from build123d import *

# Parameters (mm, degrees)
SKETCH1_W           = 65
SKETCH1_H           = 15
BOSS_EXTRUDE1_DEPTH = 4
SKETCH2_W           = 45
SKETCH2_H           = 15
BOSS_EXTRUDE2_DEPTH = 56
SKETCH3_R           = 5
CUT_EXTRUDE1_DEPTH  = 10
CUT_EXTRUDE5_REACH  = 17
BOSS_EXTRUDE3_DEPTH = 10
CUT_EXTRUDE6_REACH  = 6
SKETCH8_R           = 1.5
CUT_EXTRUDE7_DEPTH  = 22.5
SKETCH10_R          = 1.6
BOSS_EXTRUDE4_DEPTH = 20
SKETCH11_R          = 1.6
CUT_EXTRUDE8_DEPTH  = 35
SKETCH12_R          = 2.5
SKETCH12_R_2        = 1.6
BOSS_EXTRUDE5_DEPTH = 1


with BuildPart() as part:
    # Sketch1 → Boss-Extrude1 (new body)
    with BuildSketch(Plane(origin=(0, 0, 0), x_dir=(1, 0, 0), z_dir=(0, 1, 0))):
        Rectangle(SKETCH1_W, SKETCH1_H)
    extrude(amount=BOSS_EXTRUDE1_DEPTH)

    # Sketch2 → Boss-Extrude2 (add)
    with BuildSketch(Plane(origin=(0, 4, 0), x_dir=(1, 0, 0), z_dir=(0, 1, 0))):
        Rectangle(SKETCH2_W, SKETCH2_H)
    extrude(amount=BOSS_EXTRUDE2_DEPTH)

    # Sketch3 → Cut-Extrude1 (cut)
    with BuildSketch(Plane.XY.offset(7.5)):
        with Locations((0, 51)):
            Circle(SKETCH3_R)
    extrude(amount=-CUT_EXTRUDE1_DEPTH, mode=Mode.SUBTRACT)

    # Sketch6 → Cut-Extrude5 (cut, up to next)
    with BuildSketch(Plane.XY.offset(7.5), mode=Mode.PRIVATE) as cut_extrude5_sk1:
        with BuildLine():
            Line((5, 60), (22.5, 60))
            Line((22.5, 60), (22.5, 42.5))
            ThreePointArc((22.5, 42.5), (17.374368671, 54.874368671), (5, 60))
        make_face()
    cut_extrude5_tool1 = extrude(cut_extrude5_sk1.sketch, amount=-CUT_EXTRUDE5_REACH, mode=Mode.PRIVATE) & part.part
    add(cut_extrude5_tool1.solids().sort_by_distance((18.591061, 56.091061, 7.5))[0], mode=Mode.SUBTRACT)
    # Sketch6 → Cut-Extrude5 (cut, up to next)
    with BuildSketch(Plane.XY.offset(7.5), mode=Mode.PRIVATE) as cut_extrude5_sk2:
        with BuildLine():
            Line((-22.5, 42.5), (-22.5, 60))
            Line((-22.5, 60), (-5, 60))
            ThreePointArc((-5, 60), (-17.374368671, 54.874368671), (-22.5, 42.5))
        make_face()
    cut_extrude5_tool2 = extrude(cut_extrude5_sk2.sketch, amount=-CUT_EXTRUDE5_REACH, mode=Mode.PRIVATE) & part.part
    add(cut_extrude5_tool2.solids().sort_by_distance((-18.591061, 56.091061, 7.5))[0], mode=Mode.SUBTRACT)

    # Sketch7 → Boss-Extrude3 (add)
    with BuildSketch(Plane(origin=(0, 0, -7.5), x_dir=(-1, 0, 0), z_dir=(0, 0, -1))):
        with BuildLine():
            Line((-22.5, 42.5), (-22.5, 4))
            Line((-22.5, 4), (-32.5, 4))
            Line((-32.5, 4), (-32.5, 0))
            Line((-32.5, 0), (32.5, 0))
            Line((32.5, 0), (32.5, 4))
            Line((32.5, 4), (22.5, 4))
            Line((22.5, 4), (22.5, 42.5))
            ThreePointArc((22.5, 42.5), (17.374368671, 54.874368671), (5, 60))
            Line((5, 60), (-5, 60))
            ThreePointArc((-5, 60), (-17.374368671, 54.874368671), (-22.5, 42.5))
        make_face()
    extrude(amount=BOSS_EXTRUDE3_DEPTH)

    # Sketch8 → Cut-Extrude6 (cut, up to next)
    with BuildSketch(Plane(origin=(0, 4, 0), x_dir=(1, 0, 0), z_dir=(0, 1, 0)), mode=Mode.PRIVATE) as cut_extrude6_sk1:
        with Locations((-27.5, -2.5)):
            Circle(SKETCH8_R)
    cut_extrude6_tool1 = extrude(cut_extrude6_sk1.sketch, amount=-CUT_EXTRUDE6_REACH, mode=Mode.PRIVATE) & part.part
    add(cut_extrude6_tool1.solids().sort_by_distance((-27.5, 4, 2.5))[0], mode=Mode.SUBTRACT)
    # Sketch8 → Cut-Extrude6 (cut, up to next)
    with BuildSketch(Plane(origin=(0, 4, 0), x_dir=(1, 0, 0), z_dir=(0, 1, 0)), mode=Mode.PRIVATE) as cut_extrude6_sk2:
        with Locations((-27.5, 12.5)):
            Circle(SKETCH8_R)
    cut_extrude6_tool2 = extrude(cut_extrude6_sk2.sketch, amount=-CUT_EXTRUDE6_REACH, mode=Mode.PRIVATE) & part.part
    add(cut_extrude6_tool2.solids().sort_by_distance((-27.5, 4, -12.5))[0], mode=Mode.SUBTRACT)
    # Sketch8 → Cut-Extrude6 (cut, up to next)
    with BuildSketch(Plane(origin=(0, 4, 0), x_dir=(1, 0, 0), z_dir=(0, 1, 0)), mode=Mode.PRIVATE) as cut_extrude6_sk3:
        with Locations((27.5, 12.5)):
            Circle(SKETCH8_R)
    cut_extrude6_tool3 = extrude(cut_extrude6_sk3.sketch, amount=-CUT_EXTRUDE6_REACH, mode=Mode.PRIVATE) & part.part
    add(cut_extrude6_tool3.solids().sort_by_distance((27.5, 4, -12.5))[0], mode=Mode.SUBTRACT)
    # Sketch8 → Cut-Extrude6 (cut, up to next)
    with BuildSketch(Plane(origin=(0, 4, 0), x_dir=(1, 0, 0), z_dir=(0, 1, 0)), mode=Mode.PRIVATE) as cut_extrude6_sk4:
        with Locations((27.5, -2.5)):
            Circle(SKETCH8_R)
    cut_extrude6_tool4 = extrude(cut_extrude6_sk4.sketch, amount=-CUT_EXTRUDE6_REACH, mode=Mode.PRIVATE) & part.part
    add(cut_extrude6_tool4.solids().sort_by_distance((27.5, 4, 2.5))[0], mode=Mode.SUBTRACT)

    # Sketch9 → Cut-Extrude7 (cut)
    with BuildSketch(Plane(origin=(0, 60, 0), x_dir=(1, 0, 0), z_dir=(0, 1, 0))):
        Polygon((-2.875, 11.659882024), (-2.875, 17.5), (2.875, 17.5), (2.875, 11.659882024), (2.875, 8.340117976), (0, 6.680235952), (-2.875, 8.340117976), align=None)
    extrude(amount=-CUT_EXTRUDE7_DEPTH, mode=Mode.SUBTRACT)

    # Sketch10 → Boss-Extrude4 (add)
    with BuildSketch(Plane(origin=(0, 60, 0), x_dir=(1, 0, 0), z_dir=(0, 1, 0))):
        Polygon((0, 6.680235952), (2.875, 8.340117976), (2.875, 17.5), (-2.875, 17.5), (-2.875, 8.340117976), align=None)
        with Locations((0, 10)):
            Circle(SKETCH10_R, mode=Mode.SUBTRACT)
    extrude(amount=-BOSS_EXTRUDE4_DEPTH)

    # Sketch11 → Cut-Extrude8 (cut)
    with BuildSketch(Plane(origin=(0, 60, 0), x_dir=(1, 0, 0), z_dir=(0, 1, 0))):
        with Locations((0, 10)):
            Circle(SKETCH11_R)
    extrude(amount=-CUT_EXTRUDE8_DEPTH, mode=Mode.SUBTRACT)

    # Sketch12 → Boss-Extrude5 (add)
    with BuildSketch(Plane(origin=(0, 60, 0), x_dir=(1, 0, 0), z_dir=(0, 1, 0))):
        with Locations((0, 10)):
            Circle(SKETCH12_R)
        with Locations((0, 10)):
            Circle(SKETCH12_R_2, mode=Mode.SUBTRACT)
    extrude(amount=BOSS_EXTRUDE5_DEPTH)


solid = part.part
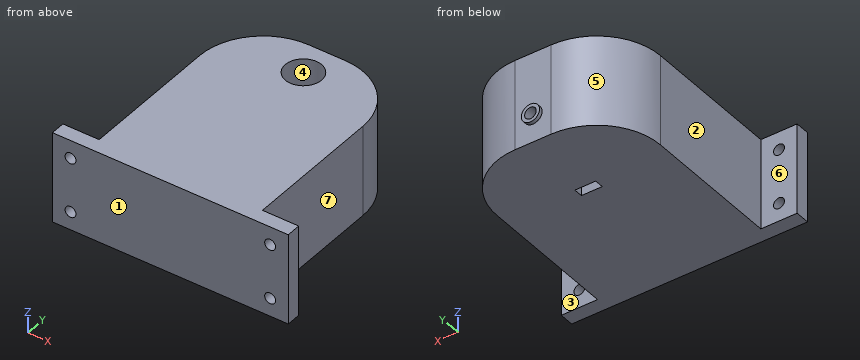
Geometry: final body of the model. Coordinates: model frame, mm. Face numbers are marked on the shaded views. A direction names the side the tool comes from. Coordinates: 2 decimals unless noted, no trailing zeros. Order: outer loops, then holes, each group sorted by start corner. A loop starts at its lowest first (then second) coordinate and runs counter-clockwise, first axis right, second up.
(1) Section query A-A (z = 2.5). Return the cut outline in (x, y).
(2) Section query D-D (z = -10). Return the cut outline in (x, y) (3 decimals), plus the area to 3 significant figures.
(3) Section query B-B (x = -27.5). Return the cut outline in (y, z), plus the area to 3 significant figures.
(4) Section query C-C (y = 51). Return the cut outline in (x, z), plus the area to 3 significant figures.
(5) Material intervals for probe 1 along Z at (x, y) = (27.5, 3.15); probe 2 along X at (y, z) = (2.45, -12.5); probe 3 along Y at (x, z) = (-0.5, -14.25), sorted ascending.
(6) Access query for the marked faces 1, 2 and 3. Directions: +Z, -Z, +X, -X, +Y, -Y. A direction counts if a zero-diameter tool reaches every point of the face in a straight line with its end or side. Return the directions, or none.
(7) First-contact query: pin 1 (4 mm diameter, centred on x = 27.5, z = -12.5, fed in from +Y); pin 2 (6 mm diameter, centred on x = -6.5, z = 2.5, fed in from +Y); pin 3 (11 mm diameter, centred on x = -25.5, z = -8, fed in from +Y). Flat tips, straight axial feed; report the tip coordinate or a pass-through.
(8) Draft query along X for the marked faces 4, 5, 6 and 7. Return one class per face: pulls with the +X half, pulls with the -X half, needs draft (parallel to the pull), parting line crosses it, or undercut.
Solution:
1. outline: (-32.5, 0) - (-29, 0) - (-29, 4) - (-32.5, 4) - close; (-26, 0) - (26, 0) - (26, 4) - (22.5, 4) - (22.5, 42.5) arc R17.5 ccw to (5, 60) - (-5, 60) arc R17.5 ccw to (-22.5, 42.5) - (-22.5, 4) - (-26, 4) - close; (29, 0) - (32.5, 0) - (32.5, 4) - (29, 4) - close; hole circle Ø10 at (0, 51)
2. outline: (-32.5, 0) - (32.5, 0) - (32.5, 4) - (22.5, 4) - (22.5, 42.5) arc R17.5 ccw to (5, 60) - (2.5, 60) - (2.5, 61) - (1.6, 61) - (1.6, 40) - (2.875, 40) - (2.875, 37.5) - (1.6, 37.5) - (1.6, 25) - (-1.6, 25) - (-1.6, 37.5) - (-2.875, 37.5) - (-2.875, 40) - (-1.6, 40) - (-1.6, 61) - (-2.5, 61) - (-2.5, 60) - (-5, 60) arc R17.5 ccw to (-22.5, 42.5) - (-22.5, 4) - (-32.5, 4) - close
2. area: 2,530 mm2
3. outline: (0, -17.5) - (4, -17.5) - (4, -14) - (0, -14) - close; (0, -11) - (4, -11) - (4, 1) - (0, 1) - close; (0, 4) - (4, 4) - (4, 7.5) - (0, 7.5) - close
3. area: 76.0 mm2
4. outline: (-20.3, -17.5) - (20.3, -17.5) - (20.3, 7.5) - (5, 7.5) - (5, -2.5) - (-5, -2.5) - (-5, 7.5) - (-20.3, 7.5) - close; hole circle Ø3.2 at (0, -10)
4. area: 907 mm2
5. probe 1: z = -17.5 to -14, -11 to 1, 4 to 7.5
5. probe 2: x = -32.5 to -29, -26 to 26, 29 to 32.5
5. probe 3: y = 0 to 37.5, 40 to 60
6. face 1: +Z, -Z, +X, -X, -Y
6. face 2: +Z, -Z, -X, +Y
6. face 3: +Z, -Z, +X, +Y
7. pin 1: stops at y = 4
7. pin 2: stops at y = 60
7. pin 3: stops at y = 51.51
8. face 4: undercut
8. face 5: pulls with the -X half
8. face 6: needs draft
8. face 7: pulls with the +X half
